Design review of the part built by this model. Coordinates are the model's own, in mm. Face numbers are marked on the shaded views. A direction names the side the tool comes from. Coordinates: 2 decimals unless noted, no trailing zeros. Order: outer loops, then holes, each group sorted by start corner. A loop starts at its lowest first (then second) coordinate and runs counter-clockwise, first axis right, second up. Notation, with made-up numbers: (15, -15.5) -> (48, -15.5) arc R21 ccw to (48, -1.5) -> close; hole circle Ø10 at (57, -25.75). An arc over 180 degrees is marked (long way). Write item = value, one per line.
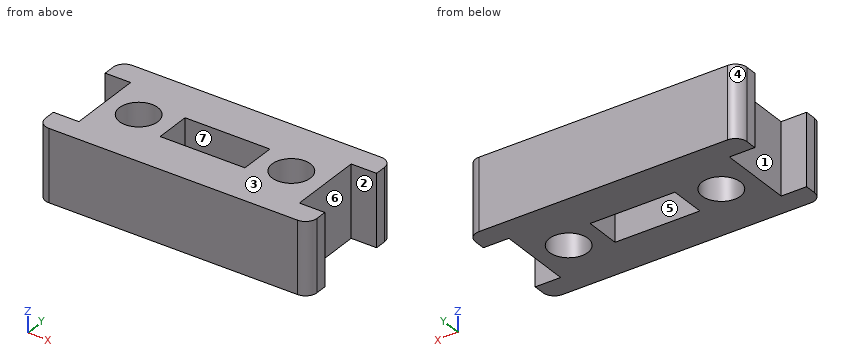
```python
from build123d import *

# Parameters (mm, degrees)
SKETCH1_W            = 7.5
SKETCH1_H            = 3.15
BOSS_EXTRUDE1_DEPTH  = 6.35
M3_CLEARANCE_HOLE1_D = 3.4
FILLET1_R            = 1


with BuildPart() as part:
    # Sketch1 → Boss-Extrude1 (new body)
    with BuildSketch(Plane.XY):
        Polygon((-12, 3.275), (-9.75, 3.275), (-9.75, -3.275), (-12, -3.275), (-12, -5.275), (12, -5.275), (12, -3.275), (9.75, -3.275), (9.75, 3.275), (12, 3.275), (12, 5.275), (-12, 5.275), align=None)
        Rectangle(SKETCH1_W, SKETCH1_H, mode=Mode.SUBTRACT)
    extrude(amount=BOSS_EXTRUDE1_DEPTH)

    # M3 Clearance Hole1 (through all)
    with Locations(Plane.XY.offset(6.35)):
        with Locations((-6.75, 0), (6.75, 0)):
            Hole(M3_CLEARANCE_HOLE1_D / 2)

    # Fillet1
    fillet1_edges = [part.edges().sort_by_distance(p)[0] for p in [
        (-12, 5.275, 3.175),
        (12, 5.275, 3.175),
        (12, -5.275, 3.175),
        (-12, -5.275, 3.175),
    ]]
    fillet(fillet1_edges, radius=FILLET1_R)


solid = part.part
```
(1) We need section C-C (y = 0). Write out the cut boundary in (x, z), and give its area (3 significant figures).
Report:
outline = (-9.75, 0) -> (-8.45, 0) -> (-8.45, 6.35) -> (-9.75, 6.35) -> close; (-5.05, 0) -> (-3.75, 0) -> (-3.75, 6.35) -> (-5.05, 6.35) -> close; (3.75, 0) -> (5.05, 0) -> (5.05, 6.35) -> (3.75, 6.35) -> close; (8.45, 0) -> (9.75, 0) -> (9.75, 6.35) -> (8.45, 6.35) -> close
area = 33.0 mm²
(2) We need section D-D (x = 6.75). Write out the cut boundary in (y, z) (3 decimals), and give its area (3 significant figures).
Report:
outline = (-5.275, 0) -> (-1.7, 0) -> (-1.7, 6.35) -> (-5.275, 6.35) -> close; (1.7, 0) -> (5.275, 0) -> (5.275, 6.35) -> (1.7, 6.35) -> close
area = 45.4 mm²
(3) We need section A-A (z = 1.75). Write out the cut boundary in (x, y) (3 decimals), and give its area (3 significant figures).
Report:
outline = (-12, -4.275) arc R1 ccw to (-11, -5.275) -> (11, -5.275) arc R1 ccw to (12, -4.275) -> (12, -3.275) -> (9.75, -3.275) -> (9.75, 3.275) -> (12, 3.275) -> (12, 4.275) arc R1 ccw to (11, 5.275) -> (-11, 5.275) arc R1 ccw to (-12, 4.275) -> (-12, 3.275) -> (-9.75, 3.275) -> (-9.75, -3.275) -> (-12, -3.275) -> close; hole circle Ø3.4 at (-6.75, 0); hole (-3.75, -1.575) -> (3.75, -1.575) -> (3.75, 1.575) -> (-3.75, 1.575) -> close; hole circle Ø3.4 at (6.75, 0)
area = 181 mm²
(4) For L1, parallel to Y at x = 6.75, z = 3.75 (3 decimals); L2, parallel to Y at x = 1.25, z = 3 (3 decimals); L3, parallel to X at y = 1, z = 1, list the stretches that pass through material, from the lowest coordinate up.
Report:
L1 = -5.275 to -1.7, 1.7 to 5.275
L2 = -5.275 to -1.575, 1.575 to 5.275
L3 = -9.75 to -8.12, -5.38 to -3.75, 3.75 to 5.38, 8.12 to 9.75
(5) The part is to be moulded in two halves that separate along X. For the marked faces 4, 5, 6 and 7, say which applies: released by +X, released by -X, zero draft, split by the parting line, or undercut.
Report:
face_4 = released by -X
face_5 = undercut
face_6 = released by +X
face_7 = undercut
(6) We need section B-B (x = 10.5). Write out the cut boundary in (y, z) (3 decimals), and give its area (3 significant figures).
Report:
outline = (-5.275, 0) -> (-3.275, 0) -> (-3.275, 6.35) -> (-5.275, 6.35) -> close; (3.275, 0) -> (5.275, 0) -> (5.275, 6.35) -> (3.275, 6.35) -> close
area = 25.4 mm²
(7) Insertion check: pin 1 (2 mm diameter, centred on x = -8, y = -3.5, fed in from -Z); pin 2 (0.9 mm diameter, centred on y = 0, z = 2, fed in from +X); pin 3 (3.5 mm diameter, centred on y = -0.5, z = 2.5, fed in from -X). Each pin has a flat end and moves straight along its axis. Give the tip position at first contact, or say it passes through.
Report:
pin_1 = 0
pin_2 = 9.75
pin_3 = -9.75
(8) For the marked faces 1, 2 and 3, list the 3-axis set-ups (+Z, -Z, +X, -X, +Y, -Y) from which the entire face can be reached by the end or side of a thin tool; tool diameter is ignored.
Report:
face_1 = +Z, -Z, -X
face_2 = +Z, -Z, +X
face_3 = +Z, +X, -X, +Y, -Y
